```python
from build123d import *

# Parameters (mm, degrees)
EXTRUDE1_DEPTH     = 5.953125
SKETCH13_R         = 7.540625
EXTRUDE3_DEPTH     = 2.4384
SKETCH2_OUTSIDE_W  = 67.282
SKETCH2_OUTSIDE_H  = 67.282
SKETCH2_OUTSIDE_R  = 5.55625
CUT_EXTRUDE1_DEPTH = 13.213179277
CUT_EXTRUDE1_DRAFT = -60
SKETCH4_R          = 3.175
CUT_EXTRUDE3_DEPTH = 13.213179277
SKETCH12_R         = 3.175
SKETCH12_R_2       = 2.350110803
EXTRUDE2_DEPTH     = 5.953125


with BuildPart() as part:
    # Sketch1 → Extrude1 (new body)
    with BuildSketch(Plane.XY):
        Polygon((0, 6.415804866), (-5.55625, 3.207902433), (-5.55625, -3.207902433), (0, -6.415804866), (5.55625, -3.207902433), (5.55625, 3.207902433), align=None)
    extrude(amount=-EXTRUDE1_DEPTH)

    # Sketch13 → Extrude3 (add)
    with BuildSketch(Plane(origin=(0, 0, -5.953125), x_dir=(-1, 0, 0), z_dir=(0, 0, -1))):
        Circle(SKETCH13_R)
    extrude(amount=-EXTRUDE3_DEPTH)


with BuildPart() as cut_extrude1_tool:
    # Sketch2 outside → Cut-Extrude1 (with draft: the straight prism first)
    with BuildSketch(Plane.XY):
        Rectangle(SKETCH2_OUTSIDE_W, SKETCH2_OUTSIDE_H)
        Circle(SKETCH2_OUTSIDE_R, mode=Mode.SUBTRACT)
    extrude(amount=-CUT_EXTRUDE1_DEPTH)
    # Cut-Extrude1: the draft: its side faces are tilted about the plane it starts from
    cut_extrude1_sides = [cut_extrude1_tool.faces().sort_by_distance(p)[0] for p in [
        (0, -33.641, -6.606589638),
        (33.641, 0, -6.606589638),
        (0, 33.641, -6.606589638),
        (-33.641, 0, -6.606589638),
        (-5.55625, 0, -6.606589638),
    ]]
    draft(cut_extrude1_sides, Plane.XY, CUT_EXTRUDE1_DRAFT)


with BuildPart() as part_1:
    add(part.part)

    # Cut-Extrude1: cut by cut_extrude1_tool
    add(cut_extrude1_tool.part, mode=Mode.SUBTRACT)

    # Sketch4 → Cut-Extrude3 (cut, through all)
    with BuildSketch(Plane.XY):
        Circle(SKETCH4_R)
    extrude(amount=-CUT_EXTRUDE3_DEPTH, mode=Mode.SUBTRACT)

    # Sketch12 → Extrude2 (add)
    with BuildSketch(Plane.XY):
        Circle(SKETCH12_R)
        Circle(SKETCH12_R_2, mode=Mode.SUBTRACT)
    extrude(amount=-EXTRUDE2_DEPTH)


solid = part_1.part
```
Could you check a few things on this model? Use its own coordinates, in mm. A direction names the side the tool comes from. Coordinates: 2 decimals unless noted, no trailing zeros. Loops run counter-clockwise (first coordinate to the right, second up) from the corner with the lowest first, then second, coordinate; pieces in that order, holes last. Notation, with made-up numbers: M -21,-0.75 L 6,-0.75 A29 ccw 6,23.25 Z; hole C 14.25,12.25 d5. An arc over 180 degrees is marked long. Put each result on its own line as item: value. Start each with the question number.
(1) For faces 1 (the face through (-2.739, 4.834, -1.733)), 2 (the face through (5.556, 0, -2)), 3 (the face through (2.739, -4.834, -1.733)), 4 (the face through (-2.8, -4.8, -1.7)), which set-ups out of +Z, -Z, +X, -X, +Y, -Y let a thin tool reach every point of the face, with its end or its side?
(2) Thinking about a two-plate mould opening in Y: for faces 5 (the face through (2.8, 4.8, -1.7)), 6 (the face through (-0.014, -5.761, -0.118)), 7 (the face through (-1.865, -1.43, -2.935)), 8 (the face through (-2, -2, -5.953)), which applies, pulls with the +Y half, pulls with the -Y half, needs draft (parallel to the pull), parting line crosses it, or undercut?
(3) Suppose I cut it at B-B on z = -3.95. Please give me the cut outline in (x, y).
(4) I need wall thicknesses on line 1 (Y direction, x = 0, z = -3.55); line 2 (Y direction, x = 1, z = -4.5); line 3 (Z direction, x = 3, y = 5.5). Which ranges of each line are inside material? Lowest first, please. Write a range as from..to.
(5) Will these pins go through, and if not, where does the flat tip stop? P1, Ø6, axis at x = 0, y = 0, coming from the +Z side; P2, Ø1, axis at y = 2.5, z = -2.5, coming from the +X side; P3, Ø2, axis at x = 3.5, z = -3.5, coming from the -Y side; P4, Ø1.5, axis at y = 5.5, z = -1, coming from the -X side.
(6) Suppose I cut it at C-C on x = -5.75. Please give me the cut outline in (y, z), then the cut area to 3 significant figures.
(7) Suppose I cut it at A-A on z = -2.5. Please give me the cut outline in (x, y).
Solutions:
1. face 1: +Z, -X, +Y
1. face 2: +Z, +X, +Y, -Y
1. face 3: +Z, +X, -Y
1. face 4: +Z, -X, -Y
2. face 5: pulls with the +Y half
2. face 6: pulls with the -Y half
2. face 7: undercut
2. face 8: needs draft
3. outline: C 0,0 d15.08; hole C 0,0 d4.7
4. line 1: y = -7.54..-2.35, 2.35..7.54
4. line 2: y = -7.47..-2.13, 2.13..7.47
4. line 3: z = -5.95..-3.51
5. P1: stops at z = 0
5. P2: stops at x = 5.56
5. P3: stops at y = -7.11
5. P4: stops at x = -2.89
6. outline: M -4.88,-5.95 L 4.88,-5.95 L 4.88,-3.51 L -4.88,-3.51 Z
6. area: 23.8 mm2
7. outline: M -5.56,-3.21 L 0,-6.42 L 5.56,-3.21 L 5.56,3.21 L 0,6.42 L -5.56,3.21 Z; hole C 0,0 d4.7
